Input: part model. Units: mm. Frame: model coordinates. A direction names the side the tool comes from. Round coordinates to 2 decimals unless told otherwise and drop trailing zeros. Loops run counter-clockwise (first coordinate to the right, second up) from the corner with the lowest first, then second, coordinate; pieces in that order, holes last. Notation, with made-up numbers: M -3,-33 L 35,-33 A19 ccw 35,-14 Z; hole C 54,-10.75 d5. An arc over 180 degrees is marked long. Put each result on its own line as item: value. Start each with the question number.
1) Pin query (flat end, axial travel): pin 1 (3 mm diameter, centred on y = -47.5, z = 7, fed in from +X); pin 2 (2.5 mm diameter, centred on x = 0, z = 6.5, fed in from -Y); pin 3 (1.8 mm diameter, centred on x = -28, z = 4.61, fed in from +Y); pin 4 (2 mm diameter, centred on y = -50, z = 2, fed in from +X). Return the tip coordinate at first contact, or that it passes through.
2) Draft query along Y for faces 1 (the face through (3, -37, 2)), 2 (the face through (-29.5, -52.95, 4.68)), 3 (the face through (3.17, -31.034, 5.07)). Return one class per face: +Y half, -Y half, draft (parallel to the pull), parting line (faces both ways), or undercut.
3) Line query: probe 1 along Z at (x, y) = (28, -52.3); probe 2 along X at (y, z) = (-41, 7.5); probe 3 along X at (y, z) = (-35, 7.25). Output: solid intervals per line, ascending.
4) Section C-C on y = -41.25. Output: boundary loops of the cut face in (x, z), plus the area to 3 significant figures.
5) Section A-A on x = -28. Output: boundary loops of the cut face in (y, z).
6) Section B-B on y = -53.5. Output: boundary loops of the cut face in (x, z).
7) Reachability of faces 4 (the face through (4, -45, 0)), 5 (the face through (-3.1, -30.98, 5.07)), 6 (the face through (-6.462, -46.784, 5.07)), 7 (the face through (26.5, -52.95, 4.68)), 8 (the face through (-4.74, -37.21, 0.99)) from +Z, -Z, +X, -X, +Y, -Y: full face, straight path, thin tool, end or side. Return the list, or none.
8) Section D-D on x = -42.5. Output: boundary loops of the cut face in (y, z).
from build123d import *

# Parameters (mm, degrees)
F1_DEPTH = 10
F2_R     = 5
F3_R     = 15
F4_R     = 1.99999
F5_R     = 1.5
F6_DEPTH = 70
F7_DEPTH = 2


# Not quite as in the source:
# - a fillet or chamfer is up to 0.001 mm smaller than in the source, because OpenCascade refuses the exact size
# - a feature names something its author has since deleted; it is built from what else it names


with BuildPart() as f1:
    # F0 (on Top) → F1 (new body)
    with BuildSketch(Plane.XY):
        with BuildLine():
            ThreePointArc((-4.8029336206, -42.6810749437), (-6.0551509394, -44.3903306382), (-7.4330361988, -46))
            Line((-7.4330361988, -46), (-2.8867513459, -46))
            Line((-2.8867513459, -46), (-3.1754264805, -45.5))
            Line((-3.1754264805, -45.5), (-3.7929698378, -44.4303835293))
            Line((-3.7929698378, -44.4303835293), (-4.8029336206, -42.6810749437))
        make_face()
        with BuildLine():
            Line((4.1882382004, -30), (0.1611781858, -30))
            ThreePointArc((0.1611781858, -30), (0.4999682243, -32.2676609927), (1.0231580796, -34.5))
            Line((1.0231580796, -34.5), (3.1754264805, -34.5))
            Line((3.1754264805, -34.5), (6.3508529611, -40))
            Line((6.3508529611, -40), (4.8029336206, -42.6810749437))
            ThreePointArc((4.8029336206, -42.6810749437), (6.0551509394, -44.3903306382), (7.4330361988, -46))
            Line((7.4330361988, -46), (8, -46))
            Line((8, -46), (8, -40.2664991614))
            ThreePointArc((8, -40.2664991614), (5.5007140279, -35.3535699402), (4.1882382004, -30))
        make_face()
        with BuildLine():
            Line((-51.8117617996, -30), (-55.8388218142, -30))
            ThreePointArc((-55.8388218142, -30), (-36.7874899568, -53.585334684), (-7.4330361988, -46))
            Line((-7.4330361988, -46), (-8, -46))
            Line((-8, -46), (-8, -40.2664991614))
            ThreePointArc((-8, -40.2664991614), (-33.4756399865, -50.367014502), (-51.8117617996, -30))
        make_face()
        with BuildLine():
            ThreePointArc((51.8117617996, -30), (33.4756399865, -50.367014502), (8, -40.2664991614))
            Line((8, -40.2664991614), (8, -46))
            Line((8, -46), (7.4330361988, -46))
            ThreePointArc((7.4330361988, -46), (36.7874899568, -53.585334684), (55.8388218142, -30))
            Line((55.8388218142, -30), (51.8117617996, -30))
        make_face()
        with BuildLine():
            ThreePointArc((-4.1882382004, -30), (-5.5007140279, -35.3535699402), (-8, -40.2664991614))
            Line((-8, -40.2664991614), (-8, -46))
            Line((-8, -46), (-7.4330361988, -46))
            ThreePointArc((-7.4330361988, -46), (-6.0551509394, -44.3903306382), (-4.8029336206, -42.6810749437))
            Line((-4.8029336206, -42.6810749437), (-6.3508529611, -40))
            Line((-6.3508529611, -40), (-3.1754264805, -34.5))
            Line((-3.1754264805, -34.5), (-1.0231580796, -34.5))
            ThreePointArc((-1.0231580796, -34.5), (-0.4999682243, -32.2676609927), (-0.1611781858, -30))
            Line((-0.1611781858, -30), (-4.1882382004, -30))
        make_face()
        with BuildLine():
            Line((1.0231580796, -34.5), (-1.0231580796, -34.5))
            ThreePointArc((-1.0231580796, -34.5), (-1.4837475224, -35.993795336), (-2.0269826837, -37.4595588572))
            ThreePointArc((-2.0269826837, -37.4595588572), (0, -36.75), (2.0269826837, -37.4595588572))
            ThreePointArc((2.0269826837, -37.4595588572), (1.4837475224, -35.993795336), (1.0231580796, -34.5))
        make_face()
        with BuildLine():
            Line((2.8867513459, -46), (7.4330361988, -46))
            ThreePointArc((7.4330361988, -46), (6.0551509394, -44.3903306382), (4.8029336206, -42.6810749437))
            Line((4.8029336206, -42.6810749437), (3.917737902, -44.2142789029))
            Line((3.917737902, -44.2142789029), (3.1754264805, -45.5))
            Line((3.1754264805, -45.5), (2.8867513459, -46))
        make_face()
        with BuildLine():
            ThreePointArc((-2.0269826837, -37.4595588572), (-1.4837475224, -35.993795336), (-1.0231580796, -34.5))
            Line((-1.0231580796, -34.5), (-3.1754264805, -34.5))
            Line((-3.1754264805, -34.5), (-6.3508529611, -40))
            Line((-6.3508529611, -40), (-4.8029336206, -42.6810749437))
            ThreePointArc((-4.8029336206, -42.6810749437), (-3.9908775438, -41.4070135311), (-3.2487256059, -40.0910051512))
            ThreePointArc((-3.2487256059, -40.0910051512), (-2.9477791452, -38.631388254), (-2.0269826837, -37.4595588572))
        make_face()
        with BuildLine():
            Line((0.1611781858, -30), (-0.1611781858, -30))
            ThreePointArc((-0.1611781858, -30), (-0.4999682243, -32.2676609927), (-1.0231580796, -34.5))
            Line((-1.0231580796, -34.5), (1.0231580796, -34.5))
            ThreePointArc((1.0231580796, -34.5), (0.4999682243, -32.2676609927), (0.1611781858, -30))
        make_face()
        with BuildLine():
            Line((3.1754264805, -34.5), (1.0231580796, -34.5))
            ThreePointArc((1.0231580796, -34.5), (1.4837475224, -35.993795336), (2.0269826837, -37.4595588572))
            ThreePointArc((2.0269826837, -37.4595588572), (2.9283266315, -38.5902471355), (3.25, -40))
            ThreePointArc((3.25, -40), (3.2496813859, -40.0455070369), (3.2487256059, -40.0910051512))
            ThreePointArc((3.2487256059, -40.0910051512), (3.9908775438, -41.4070135311), (4.8029336206, -42.6810749437))
            Line((4.8029336206, -42.6810749437), (6.3508529611, -40))
            Line((6.3508529611, -40), (3.1754264805, -34.5))
        make_face()
        with BuildLine():
            ThreePointArc((-3.2487256059, -40.0910051512), (-3.9908775438, -41.4070135311), (-4.8029336206, -42.6810749437))
            Line((-4.8029336206, -42.6810749437), (-3.7929698378, -44.4303835293))
            Line((-3.7929698378, -44.4303835293), (-3.1754264805, -45.5))
            Line((-3.1754264805, -45.5), (3.1754264805, -45.5))
            Line((3.1754264805, -45.5), (3.917737902, -44.2142789029))
            Line((3.917737902, -44.2142789029), (4.8029336206, -42.6810749437))
            ThreePointArc((4.8029336206, -42.6810749437), (3.9908775438, -41.4070135311), (3.2487256059, -40.0910051512))
            ThreePointArc((3.2487256059, -40.0910051512), (0, -43.25), (-3.2487256059, -40.0910051512))
        make_face()
        Polygon((-3.1754264805, -45.5), (-2.8867513459, -46), (2.8867513459, -46), (3.1754264805, -45.5), align=None)
    extrude(amount=F1_DEPTH)

    # F2
    f2_edges = [f1.edges().sort_by_distance(p)[0] for p in [
        (-4.188238, -30, 5),
        (4.188238, -30, 5),
    ]]
    fillet(f2_edges, radius=F2_R)

    # F3
    f3_edges = [f1.edges().sort_by_distance(p)[0] for p in [
        (-7.433036, -46, 5),
        (7.433036, -46, 5),
    ]]
    fillet(f3_edges, radius=F3_R)

    # F4 (radius 2 in the source; OpenCascade refuses exactly that, so slightly less here)
    f4_edges = [f1.edges().sort_by_distance(p)[0] for p in [
        (-55.838822, -30, 5),
        (-51.811762, -30, 5),
        (51.811762, -30, 5),
        (55.838822, -30, 5),
    ]]
    fillet(f4_edges, radius=F4_R)

    # F5 (on Front) → F6 (cut)
    with BuildSketch(Plane.XZ):
        with Locations((-28, 4.6102153137)):
            Circle(F5_R)
        with Locations((28, 4.6102153137)):
            Circle(F5_R)
    extrude(amount=F6_DEPTH, mode=Mode.SUBTRACT)

    # F0 (on Top) → F7 (cut)
    with BuildSketch(Plane.XY):
        with BuildLine():
            Line((3.1754264805, -34.5), (1.0231580796, -34.5))
            ThreePointArc((1.0231580796, -34.5), (1.4837475224, -35.993795336), (2.0269826837, -37.4595588572))
            ThreePointArc((2.0269826837, -37.4595588572), (2.9283266315, -38.5902471355), (3.25, -40))
            ThreePointArc((3.25, -40), (3.2496813859, -40.0455070369), (3.2487256059, -40.0910051512))
            ThreePointArc((3.2487256059, -40.0910051512), (3.9908775438, -41.4070135311), (4.8029336206, -42.6810749437))
            Line((4.8029336206, -42.6810749437), (6.3508529611, -40))
            Line((6.3508529611, -40), (3.1754264805, -34.5))
        make_face()
        with BuildLine():
            Line((1.0231580796, -34.5), (-1.0231580796, -34.5))
            ThreePointArc((-1.0231580796, -34.5), (-1.4837475224, -35.993795336), (-2.0269826837, -37.4595588572))
            ThreePointArc((-2.0269826837, -37.4595588572), (0, -36.75), (2.0269826837, -37.4595588572))
            ThreePointArc((2.0269826837, -37.4595588572), (1.4837475224, -35.993795336), (1.0231580796, -34.5))
        make_face()
        with BuildLine():
            ThreePointArc((-2.0269826837, -37.4595588572), (-1.4837475224, -35.993795336), (-1.0231580796, -34.5))
            Line((-1.0231580796, -34.5), (-3.1754264805, -34.5))
            Line((-3.1754264805, -34.5), (-6.3508529611, -40))
            Line((-6.3508529611, -40), (-4.8029336206, -42.6810749437))
            ThreePointArc((-4.8029336206, -42.6810749437), (-3.9908775438, -41.4070135311), (-3.2487256059, -40.0910051512))
            ThreePointArc((-3.2487256059, -40.0910051512), (-2.9477791452, -38.631388254), (-2.0269826837, -37.4595588572))
        make_face()
        with BuildLine():
            ThreePointArc((-3.2487256059, -40.0910051512), (-3.9908775438, -41.4070135311), (-4.8029336206, -42.6810749437))
            Line((-4.8029336206, -42.6810749437), (-3.7929698378, -44.4303835293))
            Line((-3.7929698378, -44.4303835293), (-3.1754264805, -45.5))
            Line((-3.1754264805, -45.5), (3.1754264805, -45.5))
            Line((3.1754264805, -45.5), (3.917737902, -44.2142789029))
            Line((3.917737902, -44.2142789029), (4.8029336206, -42.6810749437))
            ThreePointArc((4.8029336206, -42.6810749437), (3.9908775438, -41.4070135311), (3.2487256059, -40.0910051512))
            ThreePointArc((3.2487256059, -40.0910051512), (0, -43.25), (-3.2487256059, -40.0910051512))
        make_face()
    extrude(amount=F7_DEPTH, mode=Mode.SUBTRACT)


solid = f1.part
Geometry results:
1. pin 1: stops at x = 48.57
1. pin 2: stops at y = -46
1. pin 3: passes through
1. pin 4: stops at x = 45.32
2. face 1: undercut
2. face 2: draft
2. face 3: +Y half
3. probe 1: z = 0 to 3.11, 6.11 to 10
3. probe 2: x = -52.25 to -47.49, -8.51 to -3.09, 3.09 to 8.51, 47.49 to 52.25
3. probe 3: x = -54.83 to -50.63, -5.37 to 5.37, 50.63 to 54.83
4. outline: M -52.1,0 L -47.31,0 L -47.31,10 L -52.1,10 Z; M -8.69,0 L -5.63,0 L -5.63,2 L -3,2 L -3,10 L -8.69,10 Z; M 3,2 L 5.63,2 L 5.63,0 L 8.69,0 L 8.69,10 L 3,10 Z; M 47.31,0 L 52.1,0 L 52.1,10 L 47.31,10 Z
4. area: 199 mm²
5. outline: M -55,0 L -51,0 L -51,3.11 L -55,3.11 Z; M -55,6.11 L -51,6.11 L -51,10 L -55,10 Z
6. outline: M -37.04,0 L -18.96,0 L -18.96,10 L -37.04,10 Z; M 18.96,0 L 37.04,0 L 37.04,10 L 18.96,10 Z; hole C -28,4.61 d3; hole C 28,4.61 d3
7. face 4: -Z, +X, -X, +Y, -Y
7. face 5: +Z, -Z, +Y
7. face 6: +Z, -Z, -Y
7. face 7: +Y, -Y
7. face 8: -Z
8. outline: M -50.95,0 L -46.12,0 L -46.12,10 L -50.95,10 Z
